from build123d import *

# Parameters (mm, degrees)
EXTRUDE_1_DEPTH        = 5
SKETCH_2_R             = 1
EXTRUDE_2_DEPTH        = 3
HOLE_WIZARD_M2_1_D     = 1.6
HOLE_WIZARD_M2_1_DEPTH = 6
HOLE_WIZARD_M2_1_TIP   = 0.480688495


with BuildPart() as part:
    # 草图1 → 拉伸1 (new body)
    with BuildSketch(Plane.XY):
        Polygon((0.923760431, -1.6), (1.847520861, 0), (0.923760431, 1.6), (-0.923760431, 1.6), (-1.847520861, 0), (-0.923760431, -1.6), align=None)
    extrude(amount=EXTRUDE_1_DEPTH)

    # 草图2 → 拉伸2 (add)
    with BuildSketch(Plane.XY.offset(5)):
        with Locations(Location((0, 0, 0), (0, 0, 180))):
            Circle(SKETCH_2_R)
    extrude(amount=EXTRUDE_2_DEPTH)

    # M2 螺纹孔1
    with Locations(Plane(origin=(0, 0, 0), x_dir=(-1, 0, 0), z_dir=(0, 0, -1))):
        with Locations((0, 0)):
            Hole(HOLE_WIZARD_M2_1_D / 2, depth=HOLE_WIZARD_M2_1_DEPTH)
            with Locations((0, 0, -(HOLE_WIZARD_M2_1_DEPTH + HOLE_WIZARD_M2_1_TIP / 2))):  # 118° drill point
                Cone(0, HOLE_WIZARD_M2_1_D / 2, HOLE_WIZARD_M2_1_TIP, mode=Mode.SUBTRACT)


solid = part.part
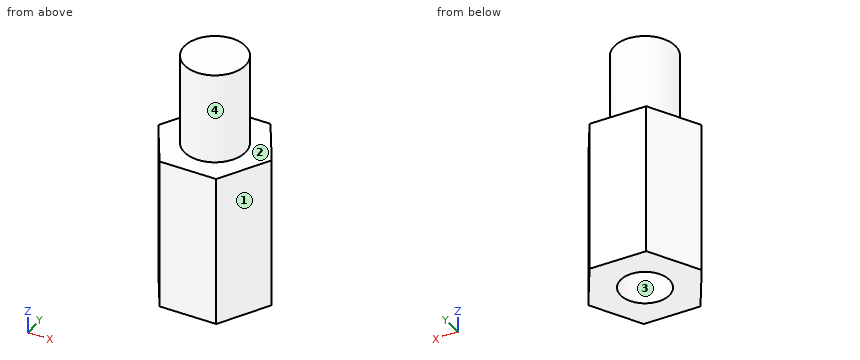
Design review of the part built by this model. Coordinates are the model's own, in mm. Face numbers are marked on the shaded views. Give positions to 0.01 mm unless a question says otherwise; leave off trailing zeros. Write each loop counter-clockwise with the first axis right and the second up, starting at its lowest first coordinate (ties: lowest second). Pieces come first, ordered by that corner, then holes. Notation, with made-up numbers: M 6,-2 L 65,-2 A13 cw 65,18 Z; hole C 44.5,68 d1. An arc over 180 degrees is marked long. Return JSON: item names as keys, results as strings. Group by question number.
Item 1: Take a section at B-B (z = 6.75). Give the boundary of the cut face in (x, y), plus the area to 3 significant figures.
Item 2: Clearance check with a flat-ended pin moving along its axis: pin 1 Ø1 at (x, z) = (0, 6.5) entering from -Y. State where the tip first meets the part, or that it passes through.
Item 3: Wall thickness on line 1 along Y through (x, z) = (0, 4.35); line 2 along Z through (x, y) = (0.7, 1.45); line 3 along Y through (x, z) = (1.3, 3): over which ranges is each line inside the solid? List them lowest first.
Item 4: Take a section at A-A (z = 2). Give the boundary of the cut face in (x, y), plus the area to 3 significant figures.
Item 5: Take a section at D-D (y = 1.2). Give the boundary of the cut face in (x, z).
Item 6: The part is to be moulded in two halves that separate along X. For the marked faces 1, 2, 3 and 4, say which applies: pulls with the +X half, pulls with the -X half, needs draft (parallel to the pull), parting line crosses it, or undercut.
Item 7: Take a section at C-C (x = -1.45). Give the boundary of the cut face in (y, z).
Return value:
{
 "1": {"outline": "C 0,0 d2", "area": "3.14 mm2"},
 "2": {"pin 1": "stops at y = -1"},
 "3": {"line 1": "y = -1.6 to -0.8, 0.8 to 1.6", "line 2": "z = 0 to 5", "line 3": "y = -0.95 to 0.95"},
 "4": {"outline": "M -1.85,0 L -0.92,-1.6 L 0.92,-1.6 L 1.85,0 L 0.92,1.6 L -0.92,1.6 Z; hole C 0,0 d1.6", "area": "6.86 mm2"},
 "5": {"outline": "M -1.15,0 L 1.15,0 L 1.15,5 L -1.15,5 Z"},
 "6": {"face 1": "pulls with the +X half", "face 2": "needs draft", "face 3": "undercut", "face 4": "parting line crosses it"},
 "7": {"outline": "M -0.69,0 L 0.69,0 L 0.69,5 L -0.69,5 Z"}
}
